```python
from build123d import *

# Parameters (mm, degrees)
SKETCH1_R           = 4.7625
BOSS_EXTRUDE1_DEPTH = 15.875
SKETCH2_W           = 0.9525
SKETCH2_H           = 1.016


with BuildPart() as part:
    # Sketch1 → Boss-Extrude1 (new body, symmetric)
    with BuildSketch(Plane.XY):
        Circle(SKETCH1_R)
    extrude(amount=BOSS_EXTRUDE1_DEPTH, both=True)

    # Sketch2 → Cut-Revolve1 (revolve, cut)
    with BuildSketch(Plane(origin=(0, 0, 0), x_dir=(1, 0, 0), z_dir=(0, 1, 0))):
        with Locations((4.28625, 10.287)):
            Rectangle(SKETCH2_W, SKETCH2_H)
        with Locations((4.28625, -10.287)):
            Rectangle(SKETCH2_W, SKETCH2_H)
    revolve(axis=Axis((0, 0, 15.875), (0, 0, -1)), mode=Mode.SUBTRACT)


solid = part.part
```
Can you work these out from the model? Positions are in its coordinate system, mm. A direction names the side the tool comes from. Give positions to 0.01 mm unless a question says otherwise; leave off trailing zeros. Order: outer loops, then holes, each group sorted by start corner. A loop starts at its lowest first (then second) coordinate and runs counter-clockwise, first axis right, second up. Notation, with made-up numbers: M 18,52 L 23,52 A20 cw 23,56 Z; hole C 23,-25 d2. An arc over 180 degrees is marked long. One line per item, written item: value.
1) We'd pull the mould along Z, two halves only. Please class faces 3 (the face through (-1, -4, 9.779)), 4 (the face through (0, 0, 15.875)), 5 (the face through (-3.78, -2.9, -13.3)): released by +Z, released by -Z, zero draft, split by the parting line, or undercut.
Answer sheet:
face 3: undercut
face 4: released by +Z
face 5: zero draft
2) I want a section at A-A, the plane y = 4.25. List the corners of the cut face in (x, z) for me (3 decimals), plus the area to 3 significant figures.
Answer sheet:
outline: M -2.149,-15.875 L 2.149,-15.875 L 2.149,-10.795 L -2.149,-10.795 Z; M -2.149,-9.779 L 2.149,-9.779 L 2.149,9.779 L -2.149,9.779 Z; M -2.149,10.795 L 2.149,10.795 L 2.149,15.875 L -2.149,15.875 Z
area: 128 mm^2
3) I want a section at D-D, the plane z = -9. List the corners of the cut face in (x, y) for me (1 decimal), plus the area to 3 significant figures.
Answer sheet:
outline: C 0,0 d9.5
area: 71.3 mm^2
4) On a 3-axis mill with a long thin cutter (end or side, diameter ignored), from which of +Z, -Z, +X, -X, +Y, -Y can I reach the whole of each face in a straight line? I mean faces 1 (the face through (-0.83, 3.72, 10.28)), 2 (the face through (0, 0, -15.875)). Say none if no direction works.
Answer sheet:
face 1: none
face 2: -Z, +X, -X, +Y, -Y
5) I want a section at B-B, the plane x = 1.5. List the corners of the cut face in (y, z) for me (3 decimals), plus the area to 3 significant figures.
Answer sheet:
outline: M -4.52,-15.875 L 4.52,-15.875 L 4.52,-10.795 L 3.502,-10.795 L 3.502,-9.779 L 4.52,-9.779 L 4.52,9.779 L 3.502,9.779 L 3.502,10.795 L 4.52,10.795 L 4.52,15.875 L -4.52,15.875 L -4.52,10.795 L -3.502,10.795 L -3.502,9.779 L -4.52,9.779 L -4.52,-9.779 L -3.502,-9.779 L -3.502,-10.795 L -4.52,-10.795 Z
area: 283 mm^2
6) I want a section at C-C, the plane y = -1.25. List the corners of the cut face in (x, z) for me (3 decimals).
Answer sheet:
outline: M -4.596,-15.875 L 4.596,-15.875 L 4.596,-10.795 L 3.599,-10.795 L 3.599,-9.779 L 4.596,-9.779 L 4.596,9.779 L 3.599,9.779 L 3.599,10.795 L 4.596,10.795 L 4.596,15.875 L -4.596,15.875 L -4.596,10.795 L -3.599,10.795 L -3.599,9.779 L -4.596,9.779 L -4.596,-9.779 L -3.599,-9.779 L -3.599,-10.795 L -4.596,-10.795 Z
7) Please list where these lines run through material, in increasing order: line 1 along Z through (x, y) = (4, 0.5) (3 decimals); line 2 along X through (y, z) = (-1.75, -12.5); line 3 along Y through (x, z) = (-0.5, 2).
Answer sheet:
line 1: z = -15.875 to -10.795, -9.779 to 9.779, 10.795 to 15.875
line 2: x = -4.43 to 4.43
line 3: y = -4.74 to 4.74
8) For P1, Ø1, axis at x = 1.5, z = -4, coming from the +Y side; P2, Ø5, axis at y = -3.5, z = -5, coming from the +X side, each with a flat end and sliding along its axis, tell me the tip position at first contact or that it passes through.
Answer sheet:
P1: stops at y = 4.66
P2: stops at x = 4.66
